Read the model definition and answer for the solid it produces. Units are mm, in the model's axes. A direction names the side the tool comes from. Coordinates: 2 decimals unless noted, no trailing zeros. Loops run counter-clockwise (first coordinate to the right, second up) from the corner with the lowest first, then second, coordinate; pieces in that order, holes last. Notation, with made-up numbers: (-1, -38) -> (4, -38) arc R23 ccw to (4, -14) -> close; hole circle Ø5 at (-7, -4.75). An arc over 180 degrees is marked (long way). Answer in a Markdown table with one row per item.
```python
from build123d import *

# Parameters (mm, degrees)
PAD_DEPTH    = 20
SKETCH001_R  = 1.5
POCKET_DEPTH = 35
PAD001_DEPTH = 5


with BuildPart() as part:
    # Sketch → Pad (new body)
    with BuildSketch(Plane.XY):
        Polygon((-55.54966, 6.705533), (-55.54966, -6.705533), (7.007378, -6.705533), (7.007378, 6.705533), (36.297374, 6.705533), (36.297374, 18.658901), (-7.007378, 18.658901), (-7.007378, 6.705533), align=None)
    extrude(amount=PAD_DEPTH)

    # Sketch001 → Pocket (cut)
    with BuildSketch(Plane.XZ):
        with Locations((26.4, 10.204084)):
            Circle(SKETCH001_R)
    extrude(amount=-POCKET_DEPTH, mode=Mode.SUBTRACT)

    # Sketch002 → Pad001 (join)
    with BuildSketch(Plane.XY.offset(7.5)):
        with BuildLine():
            add(Edge.make_bspline(
                [(-30.4665, 6.414), (-17.93, 8.30904), (-10.6414, 10.933), (-6.9843, 17.705013)],
                knots=[0, 0, 0, 0, 1, 1, 1, 1], degree=3))
            Line((-6.9843, 17.705013), (-3.352778, 3.207006))
            Line((-3.352778, 3.207006), (-29.883389, 3.207006))
            Line((-29.883389, 3.207006), (-30.4665, 6.414))
        make_face()
    extrude(amount=PAD001_DEPTH)


solid = part.part
```
1. A cutting plane is placed at D-D on y = 0. Give the vertices of the cut face in (x, z), and give its area (3 significant figures).
A:
| item | result |
|---|---|
| outline | (-55.55, 0) -> (7.01, 0) -> (7.01, 20) -> (-55.55, 20) -> close |
| area | 1,250 mm2 |
2. A tool of negligible diameter and unlimited length cuts with its end or side. For faces 1 (the flat face through (21, 6.706, 10)), 2 (the flat face through (-13, 10, 12.5)), 3 (the flat face through (-31, 6.706, 10)), from which of +Z, -Z, +X, -X, +Y, -Y can it reach the whole face along a straight path? Write none if from no direction.
A:
| item | result |
|---|---|
| face 1 | +Z, -Z, +X, -Y |
| face 2 | +Z, -X, +Y |
| face 3 | -X, +Y |
3. Given pin 1 Ø2 at (x, y) = (-12.5, 15.5) entering from -Z; pin 2 Ø3.5 at (y, z) = (15, 6.5) entering from -X; pin 3 Ø2 at (y, z) = (4, 12) entering from +X; pin 4 Ø6 at (x, z) = (14.5, 8.5) entering from -Y, each flat-ended and moving along its own axis, determine where each tip first touches the part or whether it passes through.
A:
| item | result |
|---|---|
| pin 1 | passes through |
| pin 2 | stops at x = -10.2 |
| pin 3 | stops at x = 7.01 |
| pin 4 | stops at y = 6.71 |
4. A cutting plane is placed at A-A on x = 26.4. Give the vertices of the cut face in (y, z).
A:
| item | result |
|---|---|
| outline | (6.71, 0) -> (18.66, 0) -> (18.66, 8.7) -> (6.71, 8.7) -> close; (6.71, 11.7) -> (18.66, 11.7) -> (18.66, 20) -> (6.71, 20) -> close |
5. A cutting plane is placed at B-B on z = 18. Give the vertices of the cut face in (x, y).
A:
| item | result |
|---|---|
| outline | (-55.55, -6.71) -> (7.01, -6.71) -> (7.01, 6.71) -> (36.3, 6.71) -> (36.3, 18.66) -> (-7.01, 18.66) -> (-7.01, 6.71) -> (-55.55, 6.71) -> close |
6. Find the intervals of material crossed by probe 1 along Z at (x, y) = (26.4, 14.25); probe 2 along Y at (x, z) = (-34, 2.25); probe 3 along X at (y, z) = (16.5, 2), in increasing order.
A:
| item | result |
|---|---|
| probe 1 | z = 0 to 8.7, 11.7 to 20 |
| probe 2 | y = -6.71 to 6.71 |
| probe 3 | x = -7.01 to 36.3 |
7. A cutting plane is placed at C-C on x = 10.5. Give the vertices of the cut face in (y, z).
A:
| item | result |
|---|---|
| outline | (6.71, 0) -> (18.66, 0) -> (18.66, 20) -> (6.71, 20) -> close |
